```python
from build123d import *

# Parameters (mm, degrees)
SKETCH2_W                 = 50.8
SKETCH2_H                 = 50.8
SKETCH2_W_2               = 45.72
SKETCH2_H_2               = 45.72
BOSS_EXTRUDE2_DEPTH       = 1454.15
F_97_0_5_DIAMETER_HOLE1_D = 12.7
F_97_0_5_DIAMETER_HOLE2_D = 12.7


with BuildPart() as part:
    # Sketch2 → Boss-Extrude2 (new body)
    with BuildSketch(Plane(origin=(0, 0, 0), x_dir=(1, 0, 0), z_dir=(0, 1, 0))):
        Rectangle(SKETCH2_W, SKETCH2_H)
        Rectangle(SKETCH2_W_2, SKETCH2_H_2, mode=Mode.SUBTRACT)
    extrude(amount=BOSS_EXTRUDE2_DEPTH)

    # #97 (0.5) Diameter Hole1 (through all)
    with Locations(Plane(origin=(0, 1352.55, 25.4), x_dir=(1, 0, 0), z_dir=(0, 0, 1))):
        with Locations((0, 0), (0, -1250.95)):
            Hole(F_97_0_5_DIAMETER_HOLE1_D / 2)

    # #97 (0.5) Diameter Hole2 (through all)
    with Locations(Plane(origin=(0, 822.325, 25.4), x_dir=(1, 0, 0), z_dir=(0, 0, 1))):
        with Locations((0, 0), (0, -190.5)):
            Hole(F_97_0_5_DIAMETER_HOLE2_D / 2)


solid = part.part
```
Source: CAD feature listing. Evaluate the final solid. Frame: model axes, mm. A direction names the side the tool comes from. Coordinates: 2 decimals unless noted, no trailing zeros. Loops run counter-clockwise (first coordinate to the right, second up) from the corner with the lowest first, then second, coordinate; pieces in that order, holes last. Notation, with made-up numbers: M -33.5,13.5 L -14.5,13.5 A16 cw -14.5,43.5 Z; hole C -17.5,17 d4. An arc over 180 degrees is marked long. Put each result on its own line as item: value. Start each with the question number.
1) Contact query for a flat-ended pin moving along its axis: pin 1 Ø20.5 at (x, y) = (0, 1352.55) entering from -Z. Output: stop coordinate, or through.
2) Cut plane B-B on z = -7.5. Return the cut outline in (x, y), then the cut area to 3 significant figures.
3) Reachability of faces 1 (the face through (-25.4, 717, 0)), 2 (the face through (0, 717, -22.86)) from +Z, -Z, +X, -X, +Y, -Y: full face, straight path, thin tool, end or side. Return the list, or none.
4) Pull-direction query (X, two-part tool) for faces 3 (the face through (-2, 1454.15, 24)), 4 (the face through (22.86, 717, 0)), 5 (the face through (25.4, 717, 0)), 6 (the face through (-22.86, 717, 0)); classes: pulls with the +X half, pulls with the -X half, needs draft (parallel to the pull), parting line crosses it, or undercut.
5) Cut plane A-A on y = 1155.5. Return the cut outline in (x, z).
6) Ray query, L1, parallel to Y at x = 0, z = -24.15 (3 decimals); L2, parallel to X at y = 158.5, z = -21; L3, parallel to X at y = 101, z = -24. Return the intervals inside material, ascending. Write a range as from..to.
The answers:
1. pin 1: stops at z = -25.4
2. outline: M -25.4,0 L -22.86,0 L -22.86,1454.15 L -25.4,1454.15 Z; M 22.86,0 L 25.4,0 L 25.4,1454.15 L 22.86,1454.15 Z
2. area: 7,390 mm²
3. face 1: +Z, -Z, -X, +Y, -Y
3. face 2: +Y, -Y
4. face 3: needs draft
4. face 4: undercut
4. face 5: pulls with the +X half
4. face 6: undercut
5. outline: M -25.4,-25.4 L 25.4,-25.4 L 25.4,25.4 L -25.4,25.4 Z; hole M -22.86,-22.86 L 22.86,-22.86 L 22.86,22.86 L -22.86,22.86 Z
6. L1: y = 0..95.25, 107.95..625.475, 638.175..815.975, 828.675..1346.2, 1358.9..1454.15
6. L2: x = -25.4..-22.86, 22.86..25.4
6. L3: x = -25.4..-6.32, 6.32..25.4
